Work out the finished part from the listing and answer in its coordinate system (mm). A direction names the side the tool comes from. Give positions to 0.01 mm unless a question says otherwise; leave off trailing zeros. Order: outer loops, then holes, each group sorted by start corner. A loop starts at its lowest first (then second) coordinate and runs counter-clockwise, first axis right, second up. Notation, with made-up numbers: (66.5, -39.75) - (107.5, -39.75) arc R23 ccw to (107.5, -17.75) - close; hole circle Ø10 at (46.5, 70.5). An arc over 180 degrees is marked (long way). Write each question's results on one line, items separated by ' | '.
from build123d import *

# Parameters (mm, degrees)
SKETCH1_R           = 2.5
BOSS_EXTRUDE1_DEPTH = 10


with BuildPart() as part:
    # Sketch1 → Boss-Extrude1 (new body)
    with BuildSketch(Plane(origin=(0, 0, 0), x_dir=(1, 0, 0), z_dir=(0, 1, 0))):
        with BuildLine():
            Line((-45, -35), (45, -35))
            ThreePointArc((45, -35), (52.071067812, -32.071067812), (55, -25))
            Line((55, -25), (55, 25))
            ThreePointArc((55, 25), (52.071067812, 32.071067812), (45, 35))
            Line((45, 35), (-45, 35))
            ThreePointArc((-45, 35), (-52.071067812, 32.071067812), (-55, 25))
            Line((-55, 25), (-55, -25))
            ThreePointArc((-55, -25), (-52.071067812, -32.071067812), (-45, -35))
        make_face()
        with Locations(Location((-47.8, 27.8, 0), (0, 0, 270))):
            Circle(SKETCH1_R, mode=Mode.SUBTRACT)
        with Locations(Location((-47.8, -27.8, 0), (0, 0, 90))):
            Circle(SKETCH1_R, mode=Mode.SUBTRACT)
        with Locations(Location((26.1, 30, 0), (0, 0, 270))):
            Circle(SKETCH1_R, mode=Mode.SUBTRACT)
        with Locations(Location((26.1, -30, 0), (0, 0, 90))):
            Circle(SKETCH1_R, mode=Mode.SUBTRACT)
        with BuildLine():
            Line((-30, 7.5), (30, 7.5))
            ThreePointArc((30, 7.5), (37.5, 0), (30, -7.5))
            Line((30, -7.5), (-30, -7.5))
            ThreePointArc((-30, -7.5), (-37.5, 0), (-30, 7.5))
        make_face(mode=Mode.SUBTRACT)
    extrude(amount=BOSS_EXTRUDE1_DEPTH)


solid = part.part
1. Determine the mould class of faces 3 (the face through (-1, 10, -8)), 4 (the face through (52.15, 4.93, -31.99)), 5 (the face through (-52.15, 4.93, 31.99)), 6 (the face through (26.2, 4.9, -32.5)) for opening direction Z: +Z half, -Z half, draft (parallel to the pull), parting line (faces both ways), or undercut.
Answer list:
face 3: draft | face 4: -Z half | face 5: +Z half | face 6: undercut
2. A cutting plane is placed at B-B, the plane z = 0. Write down the section's boundary in (x, y), then the cut area to 3 significant figures.
Answer list:
outline: (-55, 0) - (-37.5, 0) - (-37.5, 10) - (-55, 10) - close; (37.5, 0) - (55, 0) - (55, 10) - (37.5, 10) - close | area: 350 mm^2
3. A tool of negligible diameter and unlimited length cuts with its end or side. For faces 1 (the face through (-37.5, 4.93, 0.16)), 2 (the face through (-1, 5, 35)), from which of +Z, -Z, +X, -X, +Y, -Y can it reach the whole face along a straight path? Write none if from no direction.
Answer list:
face 1: +Y, -Y | face 2: +Z, +X, -X, +Y, -Y
4. A cutting plane is placed at D-D, the plane x = 11.5. Write down the section's boundary in (y, z), then the cut area to 3 significant figures.
Answer list:
outline: (0, -35) - (10, -35) - (10, -7.5) - (0, -7.5) - close; (0, 7.5) - (10, 7.5) - (10, 35) - (0, 35) - close | area: 550 mm^2
5. Given P1, Ø3, axis at x = -33.5, z = 2, coming from the +Y side; P2, Ø1.5, axis at y = 6.5, z = -27.5, coming from the -X side, each flat-ended and moving along its own axis, determine where each tip first touches the part or whether it passes through.
Answer list:
P1: through | P2: x = -54.85
6. A cutting plane is placed at A-A, the plane x = -47.8. Write down the section's boundary in (y, z), then the cut area to 3 significant figures.
Answer list:
outline: (0, -34.6) - (10, -34.6) - (10, -30.3) - (0, -30.3) - close; (0, -25.3) - (10, -25.3) - (10, 25.3) - (0, 25.3) - close; (0, 30.3) - (10, 30.3) - (10, 34.6) - (0, 34.6) - close | area: 592 mm^2
7. A cutting plane is placed at C-C, the plane y = 5. Write down the section's boundary in (x, z), then the cut area to 3 significant figures.
Answer list:
outline: (-55, -25) arc R10 ccw to (-45, -35) - (45, -35) arc R10 ccw to (55, -25) - (55, 25) arc R10 ccw to (45, 35) - (-45, 35) arc R10 ccw to (-55, 25) - close; hole circle Ø5 at (-47.8, -27.8); hole circle Ø5 at (-47.8, 27.8); hole (-30, -7.5) - (30, -7.5) arc R7.5 ccw to (30, 7.5) - (-30, 7.5) arc R7.5 ccw to start; hole circle Ø5 at (26.1, -30); hole circle Ø5 at (26.1, 30) | area: 6,460 mm^2
8. Straight lines are drawn through the part: line 1 (Z direction, x = 8.5, y = 9.75); line 2 (X direction, y = 9, z = 28); line 3 (Z direction, x = 26.5, y = 4). For each, find the intervals that lie inside material, in ascending order. Write a range as [from, to].
Answer list:
line 1: [-35, -7.5], [7.5, 35] | line 2: [-54.54, -50.29], [-45.31, 24.6], [27.6, 54.54] | line 3: [-35, -32.47], [-27.53, -7.5], [7.5, 27.53], [32.47, 35]
